Could you check a few things on this model? Use its own coordinates, in mm. A direction names the side the tool comes from. Coordinates: 2 decimals unless noted, no trailing zeros. Order: outer loops, then holes, each group sorted by start corner. A loop starts at its lowest first (then second) coordinate and runs counter-clockwise, first axis right, second up. Notation, with made-up numbers: (-20, 61) -> (13, 61) arc R31 ccw to (13, 91) -> close; hole circle Ø8 at (-39, 40). An arc over 180 degrees is marked (long way). Put each result on its own line as item: value. Start each with the question number.
Q1. If we section it at C-C (y = 5.5): Please give me the cut outline in (x, z).
Q2. If we section it at A-A (z = 205): Please give me the cut outline in (x, y).
Q3. Please list where these lines run through material, in increasing order: line 1 along Y through (x, z) = (-102, 81.5); line 2 along Y through (x, z) = (-107, 13); line 3 along X through (y, z) = (39.5, 44.5).
Q4. We'd pull the mould along X, two halves only. Please class faces 4 (the face through (-107.767, 66.833, 125.222)), 5 (the face through (-123.35, 93, 125)), 6 (the face through (-81.48, 56.61, 125.22)): +X half, -X half, draft (parallel to the pull), parting line (faces both ways), or undercut.
Q5. For faces 1 (the face through (-78.8, -26.6, 125.2)), 2 (the face through (-88.528, 28.018, 125.222)), 3 (the face through (-88.668, 46.121, 125.222)), which set-ups out of +Z, -Z, +X, -X, +Y, -Y let a thin tool reach every point of the face, with its end or its side?
Q6. If we section it at D-D (x = -78): Please give me the cut outline in (y, z), and give its area (3 significant figures).
Q7. If we section it at B-B (x = -109): Please give me the cut outline in (y, z).
Q8. Will these pins go through, and if not, where does the flat tip stop? pin 1 (4 mm diameter, centred on y = -8.5, z = 180.5, fed in from +X); pin 2 (1.5 mm diameter, centred on x = -119, z = 94.5, fed in from +Y); pin 3 (2 mm diameter, centred on y = 57, z = 104, fed in from +X).
from build123d import *

# Parameters (mm, degrees)
F1_DEPTH = 254
F2_DEPTH = 65.532
F3_DEPTH = 25.4


with BuildPart() as f1:
    # F0 (on Top) → F1 (new body)
    with BuildSketch(Plane.XY):
        Polygon((-40.7700149094, 2.0136271135), (-123.3497112989, 112.7550974488), (-123.3497112989, 61.7054067552), (-114.4973933697, 71.8195125399), (-100.8444875479, 61.7054067552), (-114.4973933697, 39.3378809094), (-93.5864523053, 52.7165209869), (-83.6100267408, 39.3378809094), (-93.5864523053, 16.3773968816), (-78.7674486637, 27.4278987199), (-52.8872246498, -7.2781390256), align=None)
    extrude(amount=F1_DEPTH)

    # F2 (add): a face of the model
    f2_faces = [f1.faces().sort_by_distance(p)[0] for p in [
        (-65.8273366568, 10.0748798471, 127),
    ]]
    extrude(f2_faces, amount=F2_DEPTH)

    # F3 (add): a face of the model
    f3_faces = [f1.faces().sort_by_distance(p)[0] for p in [
        (-107.6709404588, 50.5216438323, 127),
    ]]
    extrude(f3_faces, amount=F3_DEPTH)


solid = f1.part
The answers:
1. outline: (-108.17, 0) -> (-43.37, 0) -> (-43.37, 254) -> (-108.17, 254) -> close
2. outline: (-136.18, 52.57) -> (-114.5, 39.34) -> (-93.59, 52.72) -> (-83.61, 39.34) -> (-93.59, 16.38) -> (-131.3, -11.75) -> (-105.42, -46.45) -> (-52.89, -7.28) -> (-40.77, 2.01) -> (-123.35, 112.76) -> (-123.35, 73.59) -> close; hole (-115.51, 70.66) -> (-100.84, 61.71) -> (-114.5, 71.82) -> close
3. line 1: -43.9 to 10.1, 47.33 to 62.41, 62.56 to 84.12
3. line 2: -44.34 to 6.37, 44.13 to 65.46, 66.27 to 90.83
3. line 3: -114.76 to -114.24, -83.73 to -68.72
4. face 4: undercut
4. face 5: -X half
4. face 6: +X half
5. face 1: +Z, -Z, +X, -Y
5. face 2: +Z, -Z, -X
5. face 3: +Z, -Z
6. outline: (-26, 0) -> (51.94, 0) -> (51.94, 254) -> (-26, 254) -> close
6. area: 19,800 mm^2
7. outline: (-41.65, 0) -> (4.88, 0) -> (4.88, 254) -> (-41.65, 254) -> close; (42.86, 0) -> (66.68, 0) -> (66.68, 254) -> (42.86, 254) -> close; (67.75, 0) -> (93.51, 0) -> (93.51, 254) -> (67.75, 254) -> close
8. pin 1: x = -51.87
8. pin 2: y = 107.93
8. pin 3: x = -81.03
